Check sheet for the modelled part. Datum: model origin and axes. Units: mm. A direction names the side the tool comes from. Coordinates: 2 decimals unless noted, no trailing zeros. Loops run counter-clockwise (first coordinate to the right, second up) from the corner with the lowest first, then second, coordinate; pieces in that order, holes last. Notation, with made-up numbers: M 60.5,-7 L 114.5,-7 A26 ccw 114.5,21 Z; hole C 7,-18.75 d7. An arc over 180 degrees is marked long. Use CSV: the item, a comma, the result in double quotes. Start each with the question number.
(1) Section check C-C on z = -61.5. Record the cut outline in (x, y).
(2) Section check A-A on z = -110. Record the cut outline in (x, y), and give its area (3 significant figures).
(3) Draft check along X on faces 4 (the flat face through (-5, -56.5, -144)), 5 (the flat face through (-347, -45, -158)), 6 (the flat face through (347, -45, -158)), 7 (the cylindrical face through (-280.615, -24.979, -111.757)). Enter one of: pulls with the +X half, pulls with the -X half, needs draft (parallel to the pull), parting line crosses it, or undercut.
(4) Section check B-B on x = -161. Record the cut outline in (y, z), and give its area (3 significant figures).
(5) Go/stop test with flat-tipped pins: pin 1 Ø0.9 at (y, z) = (-25, -134.5) entering from -X; pin 2 Ø0.9 at (y, z) = (-25, -34) entering from +X; pin 3 Ø0.9 at (x, z) = (-99, -158.5) entering from -Y. Record where each tip stops, or that it passes through.
(6) Scan lines: line 1 (X direction, y = -24, z = -125); line 2 (Y direction, x = -380, z = -1); line 3 (Y direction, x = 140, z = -144.5). Record each from-to range of solid material in increasing order.
(7) Set-up check for faces 1 (the flat face through (-5, -42, -157)), 2 (the flat face through (-5, -23.5, -81)), 3 (the flat face through (-5, -59.5, -145)): record each of +Z, -Z, +X, -X, +Y, -Y from which the full face is reachable in a straight line by a thin tool's end or side.
from build123d import *

# Parameters (mm, degrees)
SKETCH2_W                     = 800
SKETCH2_H                     = 53
BASE_FLANGE1_DEPTH            = 3
EDGE_FLANGE1_STRIP_W          = 16
EDGE_FLANGE1_STRIP_H          = 3
EDGE_FLANGE1_STRIP_CUT_DEPTH  = 697
EDGE_FLANGE1_RELIEF_W         = 16.9
EDGE_FLANGE1_RELIEF_H         = 0.9
EDGE_FLANGE1_RELIEF_CUT_DEPTH = 3
EDGE_FLANGE1_DEPTH            = 697
EDGE_FLANGE1_FLAT_DEPTH       = 3
EDGE_FLANGE2_STRIP_W          = 16
EDGE_FLANGE2_STRIP_H          = 3
EDGE_FLANGE2_STRIP_CUT_DEPTH  = 694
EDGE_FLANGE2_DEPTH            = 694
EDGE_FLANGE3_STRIP_W          = 16
EDGE_FLANGE3_STRIP_H          = 3
EDGE_FLANGE3_STRIP_CUT_DEPTH  = 694
EDGE_FLANGE3_DEPTH            = 694
FILLET1_R                     = 10
CUT_EXTRUDE2_DEPTH            = 3
LPATTERN1_COUNT               = 4
LPATTERN1_PITCH               = 195.333333333
SKETCH20_R                    = 6
CUT_EXTRUDE3_DEPTH            = 3
SKETCH21_R                    = 6
CUT_EXTRUDE4_DEPTH            = 3
LPATTERN2_COUNT               = 5
LPATTERN2_PITCH               = 141.25
SKETCH22_R                    = 2
CUT_EXTRUDE5_DEPTH            = 3
LPATTERN3_COUNT               = 4
LPATTERN3_PITCH               = 218
SKETCH23_R                    = 13.5
CUT_EXTRUDE6_DEPTH            = 10


# Sheet-metal steps are written as plain solids
with BuildPart() as part:
    # Sketch2 → Base-Flange1 (new body)
    with BuildSketch(Plane.XY):
        Rectangle(SKETCH2_W, SKETCH2_H)
    extrude(amount=-BASE_FLANGE1_DEPTH)

    # Edge-Flange1 strip (across the edge) → Edge-Flange1 strip cut (cut)
    with BuildSketch(Plane(origin=(348.5, -26.5, -3), x_dir=(0, 1, 0), z_dir=(-1, 0, 0))):
        with Locations((-3, -1.5)):
            Rectangle(EDGE_FLANGE1_STRIP_W, EDGE_FLANGE1_STRIP_H)
    extrude(amount=EDGE_FLANGE1_STRIP_CUT_DEPTH, mode=Mode.SUBTRACT)

    # Edge-Flange1 relief (on the sheet) → Edge-Flange1 relief cut (cut)
    with BuildSketch(Plane(origin=(348.5, -21.5, -3), x_dir=(0, 1, 0), z_dir=(0, 0, -1))):
        with Locations((-7.55, 0.45)):
            Rectangle(EDGE_FLANGE1_RELIEF_W, EDGE_FLANGE1_RELIEF_H)
        with Locations((-7.55, -697.45)):
            Rectangle(EDGE_FLANGE1_RELIEF_W, EDGE_FLANGE1_RELIEF_H)
    extrude(amount=-EDGE_FLANGE1_RELIEF_CUT_DEPTH, mode=Mode.SUBTRACT)

    # Edge-Flange1 bend section (across the edge) → Edge-Flange1 (add)
    with BuildSketch(Plane(origin=(348.5, -26.5, -3), x_dir=(0, 1, 0), z_dir=(-1, 0, 0))):
        with BuildLine():
            Line((0, 2), (3, 2))
            ThreePointArc((3, 2), (3.585786438, 0.585786438), (5, 0))
            Line((5, 0), (5, -3))
            ThreePointArc((5, -3), (1.464466094, -1.535533906), (0, 2))
        make_face()
    extrude(amount=EDGE_FLANGE1_DEPTH)

    # Edge-Flange1 profile (on flange) → Edge-Flange1 flat (add)
    with BuildSketch(Plane(origin=(0, -26.5, -3), x_dir=(1, 0, 0), z_dir=(0, 1, 0))):
        Polygon((-348.5, 16.5), (-348.5, 2), (348.5, 2), (348.5, 16.5), (347, 16.5), (347, 37.5), (348.5, 37.5), (348.5, 116.5), (347, 116.5), (347, 137.5), (348.5, 137.5), (348.5, 147.5), (347, 147.5), (347, 157), (-347, 157), (-347, 147.5), (-348.5, 147.5), (-348.5, 137.5), (-347, 137.5), (-347, 116.5), (-348.5, 116.5), (-348.5, 37.5), (-347, 37.5), (-347, 16.5), align=None)
    extrude(amount=EDGE_FLANGE1_FLAT_DEPTH)

    # Edge-Flange2 strip (across the edge) → Edge-Flange2 strip cut (cut)
    with BuildSketch(Plane(origin=(-347, -26.5, -160), x_dir=(0, 0, 1), z_dir=(1, 0, 0))):
        with Locations((-3, -1.5)):
            Rectangle(EDGE_FLANGE2_STRIP_W, EDGE_FLANGE2_STRIP_H)
    extrude(amount=EDGE_FLANGE2_STRIP_CUT_DEPTH, mode=Mode.SUBTRACT)

    # Edge-Flange2 section (across the edge) → Edge-Flange2 (add)
    with BuildSketch(Plane(origin=(-347, -26.5, -160), x_dir=(0, 0, 1), z_dir=(1, 0, 0))):
        with BuildLine():
            Line((0, 2), (0, 33))
            Line((0, 33), (3, 33))
            Line((3, 33), (3, 2))
            ThreePointArc((3, 2), (3.585786438, 0.585786438), (5, 0))
            Line((5, 0), (5, -3))
            ThreePointArc((5, -3), (1.464466094, -1.535533906), (0, 2))
        make_face()
    extrude(amount=EDGE_FLANGE2_DEPTH)

    # Edge-Flange3 strip (across the edge) → Edge-Flange3 strip cut (cut)
    with BuildSketch(Plane(origin=(-347, -59.5, -157), x_dir=(0, 1, 0), z_dir=(1, 0, 0))):
        with Locations((-3, -1.5)):
            Rectangle(EDGE_FLANGE3_STRIP_W, EDGE_FLANGE3_STRIP_H)
    extrude(amount=EDGE_FLANGE3_STRIP_CUT_DEPTH, mode=Mode.SUBTRACT)

    # Edge-Flange3 section (across the edge) → Edge-Flange3 (add)
    with BuildSketch(Plane(origin=(-347, -59.5, -157), x_dir=(0, 1, 0), z_dir=(1, 0, 0))):
        with BuildLine():
            Line((0, 2), (0, 23))
            Line((0, 23), (3, 23))
            Line((3, 23), (3, 2))
            ThreePointArc((3, 2), (3.585786438, 0.585786438), (5, 0))
            Line((5, 0), (5, -3))
            ThreePointArc((5, -3), (1.464466094, -1.535533906), (0, 2))
        make_face()
    extrude(amount=EDGE_FLANGE3_DEPTH)

    # Fillet1
    fillet1_edges = [part.edges().sort_by_distance(p)[0] for p in [
        (-400, 26.5, -1.5),
        (400, 26.5, -1.5),
    ]]
    fillet(fillet1_edges, radius=FILLET1_R)

    # Sketch19 → Cut-Extrude2 (cut)
    with BuildSketch(Plane(origin=(0, 0, -160), x_dir=(-1, 0, 0), z_dir=(0, 0, -1))):
        Polygon((-286.591412012, -39.5), (-289.795706006, -33.95), (-296.204293994, -33.95), (-299.408587988, -39.5), (-296.204293994, -45.05), (-289.795706006, -45.05), align=None)
    cut_extrude2 = extrude(amount=-CUT_EXTRUDE2_DEPTH, mode=Mode.SUBTRACT)

    # LPattern1: Cut-Extrude2 ×4
    with Locations(*[(-i * LPATTERN1_PITCH, 0, 0) for i in range(1, LPATTERN1_COUNT)]):
        add(cut_extrude2, mode=Mode.SUBTRACT)

    # Sketch20 → Cut-Extrude3 (cut)
    with BuildSketch(Plane(origin=(0, 0, -3), x_dir=(-1, 0, 0), z_dir=(0, 0, -1))):
        with Locations((-380, 6.5)):
            Circle(SKETCH20_R)
        with Locations((380, 6.5)):
            Circle(SKETCH20_R)
    extrude(amount=-CUT_EXTRUDE3_DEPTH, mode=Mode.SUBTRACT)

    # Sketch21 → Cut-Extrude4 (cut)
    with BuildSketch(Plane(origin=(0, 0, -3), x_dir=(-1, 0, 0), z_dir=(0, 0, -1))):
        with Locations((-282.5, 6.5)):
            Circle(SKETCH21_R)
    cut_extrude4 = extrude(amount=-CUT_EXTRUDE4_DEPTH, mode=Mode.SUBTRACT)

    # LPattern2: Cut-Extrude4 ×5
    with Locations(*[(-i * LPATTERN2_PITCH, 0, 0) for i in range(1, LPATTERN2_COUNT)]):
        add(cut_extrude4, mode=Mode.SUBTRACT)

    # Sketch22 → Cut-Extrude5 (cut)
    with BuildSketch(Plane(origin=(0, -23.5, 0), x_dir=(1, 0, 0), z_dir=(0, 1, 0))):
        with Locations(Location((-327, 16, 0), (0, 0, 270))):
            Circle(SKETCH22_R)
        with Locations(Location((-327, 39, 0), (0, 0, 270))):
            Circle(SKETCH22_R)
        with Locations(Location((-327, 125, 0), (0, 0, 270))):
            Circle(SKETCH22_R)
    cut_extrude5 = extrude(amount=-CUT_EXTRUDE5_DEPTH, mode=Mode.SUBTRACT)

    # LPattern3: Cut-Extrude5 ×4
    with Locations(*[(i * LPATTERN3_PITCH, 0, 0) for i in range(1, LPATTERN3_COUNT)]):
        add(cut_extrude5, mode=Mode.SUBTRACT)

    # Sketch23 → Cut-Extrude6 (cut)
    with BuildSketch(Plane(origin=(0, -23.5, 0), x_dir=(1, 0, 0), z_dir=(0, 1, 0))):
        with Locations(Location((-294, 110, 0), (0, 0, 270))):
            Circle(SKETCH23_R)
    extrude(amount=-CUT_EXTRUDE6_DEPTH, mode=Mode.SUBTRACT)


solid = part.part
Outcome:
1,outline,"M -348.5,-26.5 L 348.5,-26.5 L 348.5,-23.5 L -348.5,-23.5 Z"
2,outline,"M -348.5,-26.5 L -307.5,-26.5 L -307.5,-23.5 L -348.5,-23.5 Z; M -280.5,-26.5 L 348.5,-26.5 L 348.5,-23.5 L -280.5,-23.5 Z"
2,area,"2,010 mm²"
3,face 4,"needs draft"
3,face 5,"pulls with the -X half"
3,face 6,"pulls with the +X half"
3,face 7,"undercut"
4,outline,"M -59.5,-155 A5 ccw -54.5,-160 L -28.5,-160 A5 ccw -23.5,-155 L -23.5,-5 A2 cw -21.5,-3 L 26.5,-3 L 26.5,0 L -21.5,0 A5 ccw -26.5,-5 L -26.5,-155 A2 cw -28.5,-157 L -54.5,-157 A2 cw -56.5,-155 L -56.5,-134 L -59.5,-134 Z"
4,area,"784 mm²"
5,pin 1,"stops at x = -347"
5,pin 2,"stops at x = 347"
5,pin 3,"stops at y = -58.46"
6,line 1,"x = -347 to -329, -325 to -111, -107 to 107, 111 to 325, 329 to 347"
6,line 2,"y = -26.5 to 0.5, 12.5 to 26.5"
6,line 3,"y = -59.5 to -56.5, -26.5 to -23.5"
7,face 1,"+Z, +X, -X"
7,face 2,"-Z, +X, -X, +Y"
7,face 3,"+Z, -Z, +X, -X, -Y"
